from build123d import *
from build123d.topology import SkipClean

# Parameters (mm, degrees)
SKETCH1_R           = 1.25
BOSS_EXTRUDE1_DEPTH = 15
BOSS_EXTRUDE2_START = 15
BOSS_EXTRUDE2_DEPTH = 15
SKETCH4_R           = 2.25
CUT_EXTRUDE2_DEPTH  = 2.5
SKETCH5_R           = 2.25
CUT_EXTRUDE3_DEPTH  = 2.5
SKETCH6_R           = 3.7
CUT_EXTRUDE4_DEPTH  = 2
SKETCH12_R          = 3.25
CUT_EXTRUDE5_DEPTH  = 7
SKETCH13_R          = 3.25
CUT_EXTRUDE6_DEPTH  = 7


with BuildPart() as part:
    # Sketch1 → Boss-Extrude1 (new body)
    # profile 1 of 3: a face of its own
    with BuildSketch(Plane(origin=(0, 0, 0), x_dir=(1, 0, 0), z_dir=(0, 1, 0))):
        with BuildLine():
            Line((13.265157172, 12.897160092), (13.265157172, 10.748602983))
            ThreePointArc((13.265157172, 10.748602983), (7.265157172, 1.583451593), (13.265157172, -7.581699797))
            Line((13.265157172, -7.581699797), (13.265157172, -9.730256906))
            ThreePointArc((13.265157172, -9.730256906), (17.265157172, -10.416548407), (21.265157172, -9.730256906))
            Line((21.265157172, -9.730256906), (21.265157172, -7.581699797))
            ThreePointArc((21.265157172, -7.581699797), (27.265157172, 1.583451593), (21.265157172, 10.748602983))
            Line((21.265157172, 10.748602983), (21.265157172, 12.897160092))
            ThreePointArc((21.265157172, 12.897160092), (17.265157172, 13.583451593), (13.265157172, 12.897160092))
        make_face()
        with Locations(Location((17.265157172, -3.416548407, 0), (0, 0, 270))):
            Circle(SKETCH1_R, mode=Mode.SUBTRACT)
        with Locations(Location((17.265157172, 6.583451593, 0), (0, 0, 270))):
            Circle(SKETCH1_R, mode=Mode.SUBTRACT)
        with BuildLine():
            ThreePointArc((26.432063002, 1.583451593), (24.549936544, -1.20049502), (21.265157172, -0.491281913))
            ThreePointArc((21.265157172, -0.491281913), (20.432063002, 1.583451593), (21.265157172, 3.6581851))
            ThreePointArc((21.265157172, 3.6581851), (24.549936544, 4.367398207), (26.432063002, 1.583451593))
        make_face(mode=Mode.SUBTRACT)
    # profile 2 of 3: a face of its own
    with BuildSketch(Plane(origin=(0, 0, 0), x_dir=(1, 0, 0), z_dir=(0, 1, 0))):
        with BuildLine():
            ThreePointArc((13.265157172, -7.581699797), (7.265157172, 1.583451593), (13.265157172, 10.748602983))
            Line((13.265157172, 10.748602983), (13.265157172, 12.897160092))
            ThreePointArc((13.265157172, 12.897160092), (5.265157172, 1.583451593), (13.265157172, -9.730256906))
            Line((13.265157172, -9.730256906), (13.265157172, -7.581699797))
        make_face()
    # profile 3 of 3: a face of its own
    with BuildSketch(Plane(origin=(0, 0, 0), x_dir=(1, 0, 0), z_dir=(0, 1, 0))):
        with BuildLine():
            ThreePointArc((29.265157172, 1.583451593), (27.063116143, 8.511654824), (21.265157172, 12.897160092))
            Line((21.265157172, 12.897160092), (21.265157172, 10.748602983))
            ThreePointArc((21.265157172, 10.748602983), (27.265157172, 1.583451593), (21.265157172, -7.581699797))
            Line((21.265157172, -7.581699797), (21.265157172, -9.730256906))
            ThreePointArc((21.265157172, -9.730256906), (27.063116143, -5.344751637), (29.265157172, 1.583451593))
        make_face()
    extrude(amount=BOSS_EXTRUDE1_DEPTH)

    # Sketch3 → Boss-Extrude2 (add)
    with SkipClean():  # the faces are left unmerged after this step: merging them gives an invalid solid
        with BuildSketch(Plane.XZ.offset(BOSS_EXTRUDE2_START)):
            with BuildLine():
                Line((13.265157172, -12.897160092), (13.265157172, -10.748602983))
                ThreePointArc((13.265157172, -10.748602983), (7.265157172, -1.583451593), (13.265157172, 7.581699797))
                Line((13.265157172, 7.581699797), (13.265157172, 9.730256906))
                ThreePointArc((13.265157172, 9.730256906), (5.265157172, -1.583451593), (13.265157172, -12.897160092))
            make_face()
            with BuildLine():
                Line((21.265157172, -10.748602983), (21.265157172, -12.897160092))
                ThreePointArc((21.265157172, -12.897160092), (27.063116143, -8.511654824), (29.265157172, -1.583451593))
                ThreePointArc((29.265157172, -1.583451593), (27.063116143, 5.344751637), (21.265157172, 9.730256906))
                Line((21.265157172, 9.730256906), (21.265157172, 7.581699797))
                ThreePointArc((21.265157172, 7.581699797), (27.265157172, -1.583451593), (21.265157172, -10.748602983))
            make_face()
        extrude(amount=-BOSS_EXTRUDE2_DEPTH)

    # Sketch4 → Cut-Extrude2 (cut)
    with SkipClean():  # the faces are left unmerged after this step: merging them gives an invalid solid
        with BuildSketch(Plane.XZ):
            with Locations(Location((17.265157172, -6.583451593, 0), (0, 0, 270))):
                Circle(SKETCH4_R)
        extrude(amount=-CUT_EXTRUDE2_DEPTH, mode=Mode.SUBTRACT)

    # Sketch5 → Cut-Extrude3 (cut)
    with SkipClean():  # the faces are left unmerged after this step: merging them gives an invalid solid
        with BuildSketch(Plane.XZ):
            with Locations(Location((17.265157172, 3.416548407, 0), (0, 0, 270))):
                Circle(SKETCH5_R)
        extrude(amount=-CUT_EXTRUDE3_DEPTH, mode=Mode.SUBTRACT)

    # Sketch6 → Cut-Extrude4 (cut)
    with SkipClean():  # the faces are left unmerged after this step: merging them gives an invalid solid
        with BuildSketch(Plane.XZ):
            with Locations(Location((23.432063002, -1.583451593, 0), (0, 0, 270))):
                Circle(SKETCH6_R)
        extrude(amount=-CUT_EXTRUDE4_DEPTH, mode=Mode.SUBTRACT)

    # Sketch12 → Cut-Extrude5 (cut)
    with SkipClean():  # the faces are left unmerged after this step: merging them gives an invalid solid
        with BuildSketch(Plane(origin=(0, 15, 0), x_dir=(1, 0, 0), z_dir=(0, 1, 0))):
            with Locations(Location((17.265157172, 6.583451593, 0), (0, 0, 270))):
                Circle(SKETCH12_R)
        extrude(amount=-CUT_EXTRUDE5_DEPTH, mode=Mode.SUBTRACT)

    # Sketch13 → Cut-Extrude6 (cut)
    with SkipClean():  # the faces are left unmerged after this step: merging them gives an invalid solid
        with BuildSketch(Plane(origin=(0, 15, 0), x_dir=(1, 0, 0), z_dir=(0, 1, 0))):
            with Locations(Location((17.265157172, -3.416548407, 0), (0, 0, 270))):
                Circle(SKETCH13_R)
        extrude(amount=-CUT_EXTRUDE6_DEPTH, mode=Mode.SUBTRACT)


solid = part.part
Model file for the job. Use its own axes, mm. A direction names the side the tool comes from. Give positions to 0.01 mm unless a question says otherwise; leave off trailing zeros. Order: outer loops, then holes, each group sorted by start corner. A loop starts at its lowest first (then second) coordinate and runs counter-clockwise, first axis right, second up. Notation, with made-up numbers: (-35, 78) - (15, 78) arc R21 ccw to (15, 100) - close; hole circle Ø8 at (23, -10). An arc over 180 degrees is marked (long way). Write item = value, one per line. Start each with the question number.
1. Cut at C-C, the plane y = 10.75. List the corners of the cut face in (x, z), and give its area (3 significant figures).
2. Cut at A-A, the plane y = -12.25. List the corners of the cut face in (x, z).
3. Cut at B-B, the plane z = -5.75. List the corners of the cut face in (x, y).
4. Drop flat-ended pins along their axis: P1, Ø1, axis at x = 10.5, y = -4.5, coming from the +Z side; P2, Ø3, axis at y = -5.5, z = -3.5, coming from the -X side; P3, Ø4, axis at x = 19, z = -9.5, coming from the -Y side; P4, Ø10, axis at y = -5, z = -6.5, coming from the +X side. Give the stop position or say it passes through.
5. Probe line 1 along Z through (x, y) = (17.25, 4.75); line 2 along Z through (x, y) = (17.5, 10.5); line 3 along X through (y, z) = (12.5, -7.75). List the from-to ranges inside material, lowest first.
6. Cut at D-D, the plane x = 12.5. List the corners of the cut face in (y, z).
7. Which spindle directions (+Z, -Z, +X, -X, +Y, -Y) get a long thin tool onto all of the face, cutting with end or side? Do faces 1 (the cylindrical face through (18.241, 11.549, -3.484)), 2 (the cylindrical face through (15.069, 1.232, -6.096)), 3 (the flat face through (13.265, -8, 9)), 4 (the cylindrical face through (18.32, 5.21, 4.09)), 5 (the flat face through (28, -15, -3)). Say none if no direction does.
Taken from the geometry:
q1.outline = circle Ø24 at (17.27, -1.58); hole circle Ø6.5 at (17.27, -6.58); hole circle Ø6.5 at (17.27, 3.42); hole circle Ø6 at (23.43, -1.58)
q1.area = 358 mm²
q2.outline = (13.27, -12.9) - (13.27, -10.75) arc R10 cw to (13.27, 7.58) - (13.27, 9.73) arc R12 ccw to start; (21.27, -12.9) arc R12 ccw to (21.27, 9.73) - (21.27, 7.58) arc R10 cw to (21.27, -10.75) - close
q3.outline = (6.01, -15) - (8.17, -15) - (8.17, 0) - (15.18, 0) - (15.18, 2.5) - (16.33, 2.5) - (16.33, 8) - (14.12, 8) - (14.12, 15) - (6.01, 15) - close; (18.2, 2.5) - (19.36, 2.5) - (19.36, 0) - (26.36, 0) - (26.36, -15) - (28.52, -15) - (28.52, 15) - (20.41, 15) - (20.41, 8) - (18.2, 8) - close
q4.P1 = 8.65
q4.P2 = 5.27
q4.P3 = 0
q4.P4 = 29.27
q5.line_1 = -13.58 to -7.83, -5.33 to 2.17, 4.67 to 10.42
q5.line_2 = -13.58 to -9.82, -3.34 to 0.18, 6.66 to 10.41
q5.line_3 = 6.97 to 14.23, 20.3 to 27.56
q6.outline = (-15, -12.6) - (15, -12.6) - (15, 9.43) - (-15, 9.43) - (-15, 7.21) - (0, 7.21) - (0, -10.38) - (-15, -10.38) - close
q7.face_1 = +Y
q7.face_2 = -Y
q7.face_3 = +Z, -Z, -Y
q7.face_4 = +Y, -Y
q7.face_5 = +Z, -Z, +X, -X, -Y
